Can you work these out from the model? Positions are in its coordinate system, mm. Face numbers are marked on the shaded views. A direction names the side the tool comes from. Give positions to 0.01 mm unless a question says otherwise; leave off trailing zeros. Write each loop counter-clockwise with the first axis right and the second up, starting at its lowest first coordinate (ties: lowest second). Pieces come first, ordered by that corner, then holes. Notation, with made-up numbers: (-17, 87.5) -> (-7, 87.5) arc R23 ccw to (-7, 118.5) -> close; hole circle Ø5 at (85.25, 86.25). An arc over 180 degrees is marked (long way). One line per item, written item: value.
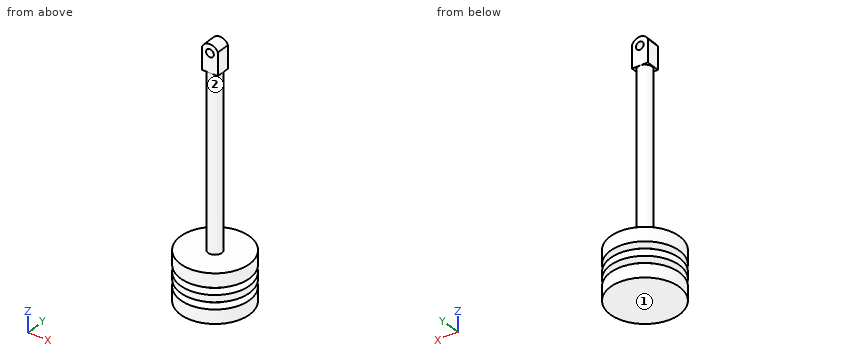
from build123d import *

# Parameters (mm, degrees)
F0_R      = 5
F1_DEPTH  = 2
F2_R      = 3.5
F3_DEPTH  = 1
F4_R      = 5
F4_R_2    = 3.5
F5_DEPTH  = 1
F6_R      = 3.5
F7_DEPTH  = 1
F8_R      = 5
F8_R_2    = 3.5
F9_DEPTH  = 2
F10_R     = 1
F11_DEPTH = 25
F13_DEPTH = 4
F15_DEPTH = 12.5
F16_R     = 0.5596686964
F17_DEPTH = 25


with BuildPart() as f1:
    # F0 (on Top) → F1 (new body)
    with BuildSketch(Plane.XY):
        Circle(F0_R)
    extrude(amount=F1_DEPTH)

    # F2 (on face) → F3 (join)
    with BuildSketch(Plane.XY.offset(2)):
        Circle(F2_R)
    extrude(amount=F3_DEPTH)

    # F4 (on face) → F5 (join)
    with BuildSketch(Plane.XY.offset(3)):
        Circle(F4_R)
        Circle(F4_R_2, mode=Mode.SUBTRACT)
        Circle(F4_R_2)
    extrude(amount=F5_DEPTH)

    # F6 (on face) → F7 (join)
    with BuildSketch(Plane.XY.offset(4)):
        Circle(F6_R)
    extrude(amount=F7_DEPTH)

    # F8 (on face) → F9 (join)
    with BuildSketch(Plane.XY.offset(5)):
        Circle(F8_R)
        Circle(F8_R_2, mode=Mode.SUBTRACT)
        Circle(F8_R_2)
    extrude(amount=F9_DEPTH)

    # F10 (on face) → F11 (join)
    with BuildSketch(Plane.XY.offset(7)):
        Circle(F10_R)
    extrude(amount=F11_DEPTH)

    # F12 (on face) → F13 (join)
    with BuildSketch(Plane.XY.offset(32)):
        with BuildLine():
            Line((1.1349343348, 1), (0, 1))
            ThreePointArc((0, 1), (0.7071067812, 0.7071067812), (1, 0))
            ThreePointArc((1, 0), (0.7071067812, -0.7071067812), (0, -1))
            Line((0, -1), (1.1349343348, -1))
            Line((1.1349343348, -1), (1.1349343348, 1))
        make_face()
        with BuildLine():
            Line((0, 1), (-1.1349343348, 1))
            Line((-1.1349343348, 1), (-1.1349343348, -1))
            Line((-1.1349343348, -1), (0, -1))
            ThreePointArc((0, -1), (-1, 0), (0, 1))
        make_face()
        with BuildLine():
            ThreePointArc((1, 0), (0.7071067812, 0.7071067812), (0, 1))
            ThreePointArc((0, 1), (-1, 0), (0, -1))
            ThreePointArc((0, -1), (0.7071067812, -0.7071067812), (1, 0))
        make_face()
    extrude(amount=F13_DEPTH)

    # F14 (on face) → F15 (intersect, symmetric)
    with BuildSketch(Plane.XZ.offset(1)):
        with BuildLine():
            Line((1.2498749086, 32), (1.2498749086, 34.7227233296))
            ThreePointArc((1.2498749086, 34.7227233296), (1.2227611454, 34.9999357877), (1.1349343348, 35.2642620149))
            Line((1.1349343348, 35.2642620149), (1.1349343348, 32))
            Line((1.1349343348, 32), (0, 32))
            Line((0, 32), (-1.1349343348, 32))
            Line((-1.1349343348, 32), (-11.0570155084, -1.4946558513))
            Line((-11.0570155084, -1.4946558513), (-0.2573039092, -3.1720956322))
            Line((-0.2573039092, -3.1720956322), (14.6179525182, 0.9926037164))
            Line((14.6179525182, 0.9926037164), (6.6368887201, 14.4441844895))
            Line((6.6368887201, 14.4441844895), (1.2498749086, 32))
        make_face()
        with BuildLine():
            Line((1.1349343348, 32), (1.1349343348, 35.2642620149))
            ThreePointArc((1.1349343348, 35.2642620149), (0, 35.9904070199), (-1.1349343348, 35.2642620149))
            Line((-1.1349343348, 35.2642620149), (-1.1349343348, 32))
            Line((-1.1349343348, 32), (0, 32))
            Line((0, 32), (1.1349343348, 32))
        make_face()
    extrude(amount=F15_DEPTH, both=True, mode=Mode.INTERSECT)

    # F16 (on face) → F17 (cut)
    with BuildSketch(Plane.XZ.offset(1)):
        with Locations((0, 34.7404070199)):
            Circle(F16_R)
    extrude(amount=-F17_DEPTH, mode=Mode.SUBTRACT)


solid = f1.part
1) For the marked faces 1 and 2, which set-ups out of +Z, -Z, +X, -X, +Y, -Y let a thin tool reach every point of the face, with its end or its side?
Answer list:
face 1: -Z, +X, -X, +Y, -Y
face 2: none
2) If we section it at B-B (y = 2): Write out the boundary of the cut face in (x, z), and give its area (3 significant figures).
Answer list:
outline: (-4.58, 0) -> (4.58, 0) -> (4.58, 2) -> (2.87, 2) -> (2.87, 3) -> (4.58, 3) -> (4.58, 4) -> (2.87, 4) -> (2.87, 5) -> (4.58, 5) -> (4.58, 7) -> (-4.58, 7) -> (-4.58, 5) -> (-2.87, 5) -> (-2.87, 4) -> (-4.58, 4) -> (-4.58, 3) -> (-2.87, 3) -> (-2.87, 2) -> (-4.58, 2) -> close
area: 57.3 mm^2
3) If we section it at D-D (x = 2.25): Write out the boundary of the cut face in (y, z).
Answer list:
outline: (-4.47, 0) -> (4.47, 0) -> (4.47, 2) -> (2.68, 2) -> (2.68, 3) -> (4.47, 3) -> (4.47, 4) -> (2.68, 4) -> (2.68, 5) -> (4.47, 5) -> (4.47, 7) -> (-4.47, 7) -> (-4.47, 5) -> (-2.68, 5) -> (-2.68, 4) -> (-4.47, 4) -> (-4.47, 3) -> (-2.68, 3) -> (-2.68, 2) -> (-4.47, 2) -> close
4) If we section it at C-C (z = 6.5): Write out the boundary of the cut face in (x, y), and give its area (3 significant figures).
Answer list:
outline: circle Ø10 at (0, 0)
area: 78.5 mm^2
5) I need wall thicknesses on L1, parallel to Z at x = 4, y = 0.5; L2, parallel to Z at x = 0, y = 0.55; L3, parallel to Z at x = 1.75, y = -1.75. Which ranges of each line are inside material? Lowest first, please.
Answer list:
L1: z = 0 to 2, 3 to 4, 5 to 7
L2: z = 0 to 34.18, 35.3 to 35.99
L3: z = 0 to 7
6) Will these pins go through, and if not, where does the flat tip stop? pin 1 (6 mm diameter, centred on x = -3.5, y = -1.5, fed in from +Z); pin 2 (1.1 mm diameter, centred on x = 0, z = 34.5, fed in from -Y); pin 3 (1 mm diameter, centred on y = 0, z = 34, fed in from +X); pin 4 (1.2 mm diameter, centred on x = 0.5, y = -0.5, fed in from -Z).
Answer list:
pin 1: stops at z = 35.87
pin 2: stops at y = -1
pin 3: stops at x = 1.13
pin 4: stops at z = 0
